from build123d import *

# Parameters (mm, degrees)
BOSS_EXTRUDE1_DEPTH = 2.54


with BuildPart() as part:
    # Sketch1 → Boss-Extrude1 (new body)
    with BuildSketch(Plane(origin=(0, 0, 0), x_dir=(1, 0, 0), z_dir=(0, 1, 0))):
        with BuildLine():
            Line((-27.94, 0), (-27.94, 25.4))
            ThreePointArc((-27.94, 25.4), (-27.196051224, 27.196051224), (-25.4, 27.94))
            Line((-25.4, 27.94), (0, 27.94))
            Line((0, 27.94), (25.4, 27.94))
            ThreePointArc((25.4, 27.94), (27.196051224, 27.196051224), (27.94, 25.4))
            Line((27.94, 25.4), (27.94, 0))
            Line((27.94, 0), (27.94, -25.4))
            ThreePointArc((27.94, -25.4), (27.196051224, -27.196051224), (25.4, -27.94))
            Line((25.4, -27.94), (0, -27.94))
            Line((0, -27.94), (-25.4, -27.94))
            ThreePointArc((-25.4, -27.94), (-27.196051224, -27.196051224), (-27.94, -25.4))
            Line((-27.94, -25.4), (-27.94, 0))
        make_face()
        with BuildLine():
            Line((-18.288, 22.86), (-18.288, -22.86))
            ThreePointArc((-18.288, -22.86), (-19.939, -24.511), (-21.59, -22.86))
            Line((-21.59, -22.86), (-21.59, 22.86))
            ThreePointArc((-21.59, 22.86), (-19.939, 24.511), (-18.288, 22.86))
        make_face(mode=Mode.SUBTRACT)
        with BuildLine():
            Line((18.288, 22.86), (18.288, -22.86))
            ThreePointArc((18.288, -22.86), (19.939, -24.511), (21.59, -22.86))
            Line((21.59, -22.86), (21.59, 22.86))
            ThreePointArc((21.59, 22.86), (19.939, 24.511), (18.288, 22.86))
        make_face(mode=Mode.SUBTRACT)
    extrude(amount=BOSS_EXTRUDE1_DEPTH)


solid = part.part
The model under review builds one solid part; all positions refer to its coordinate system, in mm. A direction names the side the tool comes from. Coordinates: 2 decimals unless noted, no trailing zeros. Write each loop counter-clockwise with the first axis right and the second up, starting at its lowest first coordinate (ties: lowest second). Pieces come first, ordered by that corner, then holes. Notation, with made-up numbers: (43, -38) - (85, -38) arc R21 cw to (85, -16) - close; hole circle Ø10 at (22, 64.25). An arc over 180 degrees is marked (long way). Answer as a JSON object with one key per item and string values. Group by question number.
1. Add section A-A (y = 0.9). Give the boundary of the cut face in (x, z).
2. Machinability: for faces 5 (the face through (0, 0, 0)), 6 (the face through (-21.59, 1, 0)), which of the approach directions +Z, -Z, +X, -X, +Y, -Y give a long, thin tool a straight path to every point of the face, cutting with its end or side? Answer none if there is none.
3. Clearance check with a flat-ended pin moving along its axis: pin 1 Ø1 at (x, z) = (-5, 7) entering from -Y. State where the tip first meets the part, or that it passes through.
4. Add section B-B (z = 19). Give the boundary of the cut face in (x, y), plus the area to 3 significant figures.
5. Mouldability with a two-part tool opening along X and no side actions: class faces 1 (the face through (-18.288, 1, 0)), 2 (the face through (27.176, 1.252, -27.216)), 3 (the face through (0, 2.54, 0)), 4 (the face through (-19.9, 1.25, 24.51)) as pulls with the +X half, pulls with the -X half, needs draft (parallel to the pull), parting line crosses it, or undercut.
6. To check wall thickness, follow probe 1 along X at (y, z) = (1.3, 11); probe 2 along Z at (x, y) = (25.5, 0.5); probe 3 along Z at (x, y) = (21, 0.3). State the ranges of each line that lie inside material, in increasing order.
Findings:
{
 "1": {"outline": "(-27.94, -25.4) arc R2.54 ccw to (-25.4, -27.94) - (25.4, -27.94) arc R2.54 ccw to (27.94, -25.4) - (27.94, 25.4) arc R2.54 ccw to (25.4, 27.94) - (-25.4, 27.94) arc R2.54 ccw to (-27.94, 25.4) - close; hole (-21.59, -22.86) arc R1.65 ccw to (-18.29, -22.86) - (-18.29, 22.86) arc R1.65 ccw to (-21.59, 22.86) - close; hole (18.29, -22.86) arc R1.65 ccw to (21.59, -22.86) - (21.59, 22.86) arc R1.65 ccw to (18.29, 22.86) - close"},
 "2": {"face 5": "+Z, -Z, +X, -X, -Y", "face 6": "+Y, -Y"},
 "3": {"pin 1": "y = 0"},
 "4": {"outline": "(-27.94, 0) - (-21.59, 0) - (-21.59, 2.54) - (-27.94, 2.54) - close; (-18.29, 0) - (18.29, 0) - (18.29, 2.54) - (-18.29, 2.54) - close; (21.59, 0) - (27.94, 0) - (27.94, 2.54) - (21.59, 2.54) - close", "area": "125 mm²"},
 "5": {"face 1": "undercut", "face 2": "pulls with the +X half", "face 3": "needs draft", "face 4": "undercut"},
 "6": {"probe 1": "-27.94 to -21.59, -18.29 to 18.29, 21.59 to 27.94", "probe 2": "-27.94 to 27.94", "probe 3": "-27.94 to -24.12, 24.12 to 27.94"}
}
